Can you work these out from the model? Positions are in its coordinate system, mm. Face numbers are marked on the shaded views. A direction names the side the tool comes from. Coordinates: 2 decimals unless noted, no trailing zeros. Order: outer loops, then holes, each group sorted by start corner. A loop starts at its lowest first (then second) coordinate and runs counter-clockwise, first axis right, second up. Notation, with made-up numbers: (32, 17.25) -> (68, 17.25) arc R18 cw to (68, 44.25) -> close; hole circle Ø1 at (25.5, -25). An arc over 180 degrees is marked (long way). Answer in a Markdown table with one row per item. Add a question column.
1. If I drill on line 1 along X through (y, z) = (-8.25, 5.5); line 2 along Z through (x, y) = (6.25, -2.25); line 3 along Z through (x, y) = (-1, -4), over which ranges is the centre line in solid material (lowest first)? Write a range as [from, to].
2. Imagine slicing it at D-D on z = 16. Write out the boundary of the cut face in (x, y), plus the area to 3 significant figures.
3. On a 3-axis mill with a long thin cutter (end or side, diameter ignored), from which of +Z, -Z, +X, -X, +Y, -Y can I reach the whole of each face in a straight line? I mean the marked faces 4, 5 and 6. Say none if no direction works.
4. Imagine slicing it at B-B on z = 10.5. Write out the boundary of the cut face in (x, y), plus the area to 3 significant figures.
5. Imagine slicing it at A-A on x = 0. State how many separate pieces and enclosed holes the cut face has, plus the area to 3 significant figures.
6. Imagine slicing it at C-C on y = -0.5. Write out the boundary of the cut face in (x, z), plus the area to 3 significant figures.
7. We'd pull the mould along X, two halves only. Please class the marked faces 1, 2 and 3: pulls with the +X half, pulls with the -X half, needs draft (parallel to the pull), parting line crosses it, or undercut.
8. Will these pins go through, and if not, where does the flat tip stop? pin 1 (6 mm diameter, centred on x = 3.5, z = 12.5, fed in from -Y); pin 2 (10 mm diameter, centred on x = -4.5, y = -10, fed in from -Z); pin 3 (1 mm diameter, centred on x = 6, z = 2, fed in from +Y).
from build123d import *

# Parameters (mm, degrees)
BOSS_EXTRUDE1_DEPTH = 10
SKETCH2_W           = 17
SKETCH2_H           = 17
CUT_EXTRUDE1_DEPTH  = 6
CUT_EXTRUDE2_DEPTH  = 3
BOSS_EXTRUDE2_DEPTH = 1


with BuildPart() as part:
    # Sketch1 → Boss-Extrude1 (new body, symmetric)
    with BuildSketch(Plane(origin=(0, 0, 0), x_dir=(0, 0, -1), z_dir=(1, 0, 0))):
        Polygon((0, 0), (-20, 0), (-20, -3), (-11.5, -11.5), (-3, -20), (0, -20), align=None)
    extrude(amount=BOSS_EXTRUDE1_DEPTH, both=True)

    # Sketch2 → Cut-Extrude1 (cut, symmetric)
    with BuildSketch(Plane(origin=(0, 0, 0), x_dir=(0, 0, -1), z_dir=(1, 0, 0))):
        with Locations((-11.5, -11.5)):
            Rectangle(SKETCH2_W, SKETCH2_H)
    extrude(amount=CUT_EXTRUDE1_DEPTH, both=True, mode=Mode.SUBTRACT)

    # Sketch3 → Cut-Extrude2 (cut)
    with BuildSketch(Plane.XY.offset(3)):
        with BuildLine():
            Line((-3, -9), (-3, -12))
            ThreePointArc((-3, -12), (0, -15), (3, -12))
            Line((3, -12), (3, -9))
            ThreePointArc((3, -9), (0, -6), (-3, -9))
        make_face()
    cut_extrude2 = extrude(amount=-CUT_EXTRUDE2_DEPTH, mode=Mode.SUBTRACT)

    # Sketch4 → Boss-Extrude2 (add)
    with BuildSketch(Plane(origin=(0, 0, 0), x_dir=(-1, 0, 0), z_dir=(0, 0, -1))):
        with BuildLine():
            Line((-1, -3), (1, -3))
            ThreePointArc((1, -3), (1.85, -2.15), (1, -1.3))
            Line((1, -1.3), (-1, -1.3))
            ThreePointArc((-1, -1.3), (-1.85, -2.15), (-1, -3))
        make_face()
        with BuildLine():
            Line((-1, -18.3), (1, -18.3))
            ThreePointArc((1, -18.3), (1.85, -17.45), (1, -16.6))
            Line((1, -16.6), (-1, -16.6))
            ThreePointArc((-1, -16.6), (-1.85, -17.45), (-1, -18.3))
        make_face()
    boss_extrude2 = extrude(amount=BOSS_EXTRUDE2_DEPTH)

    # Mirror1: Cut-Extrude2, Boss-Extrude2 across plane
    add(cut_extrude2.mirror(Plane(origin=(0, 0, 0), x_dir=(0, -0.707106781, 0.707106781), z_dir=(0, 0.707106781, 0.707106781))), mode=Mode.SUBTRACT)
    add(boss_extrude2.mirror(Plane(origin=(0, 0, 0), x_dir=(0, -0.707106781, 0.707106781), z_dir=(0, 0.707106781, 0.707106781))))


solid = part.part
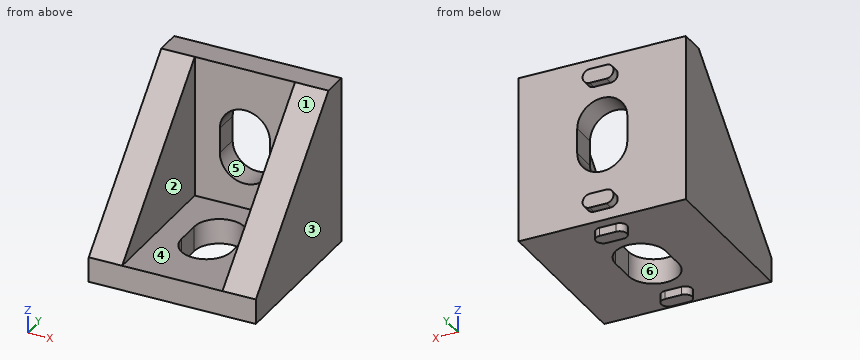
Answers follow:
| question | item | result |
|---|---|---|
| 1 | line 1 | x = [-10, -6], [6, 10] |
| 1 | line 2 | z = [0, 20] |
| 1 | line 3 | z = [0, 3] |
| 2 | outline | (-10, -7) -> (-6, -7) -> (-6, -3) -> (6, -3) -> (6, -7) -> (10, -7) -> (10, 0) -> (-10, 0) -> close |
| 2 | area | 92.0 mm² |
| 3 | face 4 | +Z, -Y |
| 3 | face 5 | +Y, -Y |
| 3 | face 6 | +Z, -Z |
| 4 | outline | (-10, -12.5) -> (-6, -12.5) -> (-6, -3) -> (-3, -3) -> (-3, 0) -> (-10, 0) -> close; (3, -3) -> (6, -3) -> (6, -12.5) -> (10, -12.5) -> (10, 0) -> (3, 0) -> close |
| 4 | area | 118 mm² |
| 5 | separate pieces | 3 |
| 5 | enclosed holes | 0 |
| 5 | area | 63.8 mm² |
| 6 | outline | (-10, 0) -> (10, 0) -> (10, 20) -> (-10, 20) -> close; hole (-3, 9) arc R3 ccw to (3, 9) -> (3, 12) arc R3 ccw to (-3, 12) -> close |
| 6 | area | 354 mm² |
| 7 | face 1 | needs draft |
| 7 | face 2 | undercut |
| 7 | face 3 | pulls with the +X half |
| 8 | pin 1 | stops at y = -12.16 |
| 8 | pin 2 | stops at z = 0 |
| 8 | pin 3 | stops at y = 0 |
